Can you work these out from the model? Positions are in its coordinate system, mm. A direction names the side the tool comes from. Coordinates: 2 decimals unless noted, no trailing zeros. Loops run counter-clockwise (first coordinate to the right, second up) from the corner with the lowest first, then second, coordinate; pieces in that order, holes last.
```python
from build123d import *

# Parameters (mm, degrees)
SKETCH1_W                        = 1206.5
SKETCH1_H                        = 596.9
SKETCH1_W_2                      = 1201.42
SKETCH1_H_2                      = 591.82
BOSS_EXTRUDE1_DEPTH              = 177.8
SKETCH2_W                        = 1206.5
SKETCH2_H                        = 596.9
BOSS_EXTRUDE2_DEPTH              = 2.54
FILLET1_R                        = 50.8
F_7_8_0_875_DIAMETER_HOLE1_D     = 22.225
F_7_8_0_875_DIAMETER_HOLE1_DEPTH = 2.54


with BuildPart() as part:
    # Sketch1 → Boss-Extrude1 (new body)
    with BuildSketch(Plane(origin=(0, 0, 0), x_dir=(1, 0, 0), z_dir=(0, 1, 0))):
        Rectangle(SKETCH1_W, SKETCH1_H)
        Rectangle(SKETCH1_W_2, SKETCH1_H_2, mode=Mode.SUBTRACT)
    extrude(amount=BOSS_EXTRUDE1_DEPTH)

    # Sketch2 → Boss-Extrude2 (add)
    with BuildSketch(Plane.XZ):
        Rectangle(SKETCH2_W, SKETCH2_H)
    extrude(amount=BOSS_EXTRUDE2_DEPTH)

    # Fillet1
    fillet1_edges = [part.edges().sort_by_distance(p)[0] for p in [
        (600.71, 88.9, 295.91),
        (600.71, 88.9, -295.91),
        (-600.71, 88.9, -295.91),
        (-600.71, 88.9, 295.91),
        (603.25, 87.63, 298.45),
        (-603.25, 87.63, 298.45),
        (-603.25, 87.63, -298.45),
        (603.25, 87.63, -298.45),
    ]]
    fillet(fillet1_edges, radius=FILLET1_R)

    # 7/8 (0.875) Diameter Hole1
    with Locations(Plane(origin=(0, 0, 0), x_dir=(1, 0, 0), z_dir=(0, 1, 0))):
        with Locations((575.31, 0), (-575.31, 0)):
            Hole(F_7_8_0_875_DIAMETER_HOLE1_D / 2, depth=F_7_8_0_875_DIAMETER_HOLE1_DEPTH)


solid = part.part
```
Item 1: Suppose I cut it at A-A, the plane y = 22. Please give me the cut outline in (x, z).
Results are:
outline: (-603.25, -247.65) arc R50.8 ccw to (-552.45, -298.45) - (552.45, -298.45) arc R50.8 ccw to (603.25, -247.65) - (603.25, 247.65) arc R50.8 ccw to (552.45, 298.45) - (-552.45, 298.45) arc R50.8 ccw to (-603.25, 247.65) - close; hole (-600.71, -245.11) arc R50.8 ccw to (-549.91, -295.91) - (549.91, -295.91) arc R50.8 ccw to (600.71, -245.11) - (600.71, 245.11) arc R50.8 ccw to (549.91, 295.91) - (-549.91, 295.91) arc R50.8 ccw to (-600.71, 245.11) - close
Item 2: On a 3-axis mill with a long thin cutter (end or side, diameter ignored), from which of +Z, -Z, +X, -X, +Y, -Y can I reach the whole of each face in a straight line? I mean faces 1 (the face through (-586.224, 90.145, -280.634)), 2 (the face through (-8, -2.54, 4)). Say none if no direction works.
Results are:
face 1: +Y
face 2: +Z, -Z, +X, -X, -Y
Item 3: Suppose I cut it at C-C, the plane x = -575.31. Please give me the cut outline in (y, z), plus the area to 3 significant figures.
Results are:
outline: (-2.54, -293.02) - (177.8, -293.02) - (177.8, -289.1) - (0, -289.1) - (0, -11.11) - (-2.54, -11.11) - close; (-2.54, 11.11) - (0, 11.11) - (0, 289.1) - (177.8, 289.1) - (177.8, 293.02) - (-2.54, 293.02) - close
area: 2,820 mm2
Item 4: Suppose I cut it at D-D, the plane z = -90. Please give me the cut outline in (x, y), plus the area to 3 significant figures.
Results are:
outline: (-603.25, -2.54) - (603.25, -2.54) - (603.25, 177.8) - (600.71, 177.8) - (600.71, 0) - (-600.71, 0) - (-600.71, 177.8) - (-603.25, 177.8) - close
area: 3,970 mm2
Item 5: I need wall thicknesses on line 1 along Z through (x, y) = (-428, 162); line 2 along X through (y, z) = (156, 165); line 3 along Y through (x, z) = (521.5, 249.5). Which ranges of each line are inside material? Lowest first, please.
Results are:
line 1: z = -298.45 to -295.91, 295.91 to 298.45
line 2: x = -603.25 to -600.71, 600.71 to 603.25
line 3: y = -2.54 to 0
Item 6: Suppose I cut it at B-B, the plane z = 0. Please give me the cut outline in (x, y), plus the area to 3 significant figures.
Results are:
outline: (-603.25, -2.54) - (-586.42, -2.54) - (-586.42, 0) - (-600.71, 0) - (-600.71, 177.8) - (-603.25, 177.8) - close; (-564.2, -2.54) - (564.2, -2.54) - (564.2, 0) - (-564.2, 0) - close; (586.42, -2.54) - (603.25, -2.54) - (603.25, 177.8) - (600.71, 177.8) - (600.71, 0) - (586.42, 0) - close
area: 3,850 mm2
Item 7: I'm going to push flat-ended pins straight in: P1, Ø5, axis at x = -349.5, z = 233.5, coming from the +Y side; P2, Ø20, axis at x = 575.31, z = 0, coming from the +Y side. Where does each tip first touch, or does it pass through?
Results are:
P1: stops at y = 0
P2: passes through
